```python
from build123d import *

# Parameters (mm, degrees)
SKETCH1_W           = 91.44
SKETCH1_H           = 152.4
BOSS_EXTRUDE1_DEPTH = 1.6
CUT_EXTRUDE1_REACH  = 90.878
SKETCH2_R           = 1.75
SKETCH3_W           = 91.44
SKETCH3_H           = 3
CUT_EXTRUDE2_DEPTH  = 0.0001


with BuildPart() as part:
    # Sketch1 → Boss-Extrude1 (new body)
    with BuildSketch(Plane(origin=(0, 0, 0), x_dir=(1, 0, 0), z_dir=(0, 1, 0))):
        Rectangle(SKETCH1_W, SKETCH1_H)
    extrude(amount=BOSS_EXTRUDE1_DEPTH)

    # Sketch2 → Cut-Extrude1 (cut, up to next)
    with BuildSketch(Plane(origin=(0, 1.6, 0), x_dir=(1, 0, 0), z_dir=(0, 1, 0)), mode=Mode.PRIVATE) as cut_extrude1_sk1:
        with Locations(Location((-38.22, 70.2, 0), (0, 0, 270))):
            Circle(SKETCH2_R)
    cut_extrude1_tool1 = extrude(cut_extrude1_sk1.sketch, amount=-CUT_EXTRUDE1_REACH, mode=Mode.PRIVATE) & part.part
    # Sketch2 → Cut-Extrude1 (cut, up to next)
    with BuildSketch(Plane(origin=(0, 1.6, 0), x_dir=(1, 0, 0), z_dir=(0, 1, 0)), mode=Mode.PRIVATE) as cut_extrude1_sk2:
        with Locations(Location((-33.72, -70.2, 0), (0, 0, 270))):
            Circle(SKETCH2_R)
    cut_extrude1_tool2 = extrude(cut_extrude1_sk2.sketch, amount=-CUT_EXTRUDE1_REACH, mode=Mode.PRIVATE) & part.part
    # Sketch2 → Cut-Extrude1 (cut, up to next)
    with BuildSketch(Plane(origin=(0, 1.6, 0), x_dir=(1, 0, 0), z_dir=(0, 1, 0)), mode=Mode.PRIVATE) as cut_extrude1_sk3:
        with Locations(Location((35.72, -70.2, 0), (0, 0, 270))):
            Circle(SKETCH2_R)
    cut_extrude1_tool3 = extrude(cut_extrude1_sk3.sketch, amount=-CUT_EXTRUDE1_REACH, mode=Mode.PRIVATE) & part.part
    # Sketch2 → Cut-Extrude1 (cut, up to next)
    with BuildSketch(Plane(origin=(0, 1.6, 0), x_dir=(1, 0, 0), z_dir=(0, 1, 0)), mode=Mode.PRIVATE) as cut_extrude1_sk4:
        with Locations(Location((13.78, 70.2, 0), (0, 0, 270))):
            Circle(SKETCH2_R)
    cut_extrude1_tool4 = extrude(cut_extrude1_sk4.sketch, amount=-CUT_EXTRUDE1_REACH, mode=Mode.PRIVATE) & part.part
    add(cut_extrude1_tool1.solids().sort_by_distance((-38.22, 1.6, -70.2))[0], mode=Mode.SUBTRACT)
    add(cut_extrude1_tool2.solids().sort_by_distance((-33.72, 1.6, 70.2))[0], mode=Mode.SUBTRACT)
    add(cut_extrude1_tool3.solids().sort_by_distance((35.72, 1.6, 70.2))[0], mode=Mode.SUBTRACT)
    add(cut_extrude1_tool4.solids().sort_by_distance((13.78, 1.6, -70.2))[0], mode=Mode.SUBTRACT)

    # Sketch3 → Cut-Extrude2 (cut)
    with BuildSketch(Plane(origin=(0, 1.6, 0), x_dir=(1, 0, 0), z_dir=(0, 1, 0))):
        with Locations((0, 74.7)):
            Rectangle(SKETCH3_W, SKETCH3_H)
        with Locations((0, -74.7)):
            Rectangle(SKETCH3_W, SKETCH3_H)
    extrude(amount=-CUT_EXTRUDE2_DEPTH, mode=Mode.SUBTRACT)


solid = part.part
```
Source: CAD feature listing. Evaluate the final solid. Frame: model axes, mm. Coordinates: 2 decimals unless noted, no trailing zeros. Write each loop counter-clockwise with the first axis right and the second up, starting at its lowest first coordinate (ties: lowest second). Pieces come first, ordered by that corner, then holes. Notation, with made-up numbers: (72, 83) - (108, 83) arc R23 ccw to (108, 102) - close; hole circle Ø1 at (3, 46). An arc over 180 degrees is marked (long way). Answer as a JSON object with one key per item and string values.
Q1. Draft query along Z for faces 1 (the flat face through (-1, 1.6, 75)), 2 (the cylindrical face through (13.86, 0.81, -71.95)), 3 (the cylindrical face through (34.01, 0.81, 69.82)). Return one class per face: released by +Z, released by -Z, zero draft, split by the parting line, or undercut.
Ans:
{"face 1": "zero draft", "face 2": "undercut", "face 3": "undercut"}
Q2. Section query B-B, the plane z = 70.2. Output: boundary loops of the cut face in (x, y), plus the area to 3 significant figures.
Ans:
{"outline": "(-45.72, 0) - (-35.47, 0) - (-35.47, 1.6) - (-45.72, 1.6) - close; (-31.97, 0) - (33.97, 0) - (33.97, 1.6) - (-31.97, 1.6) - close; (37.47, 0) - (45.72, 0) - (45.72, 1.6) - (37.47, 1.6) - close", "area": "135 mm2"}
Q3. First-contact query: pin 1 Ø4 at (x, z) = (13.78, -70.2) entering from +Y; pin 2 Ø3 at (x, z) = (-33.72, 70.2) entering from -Y. Flat tips, straight axial feed; report the tip coordinate or a pass-through.
Ans:
{"pin 1": "stops at y = 1.6", "pin 2": "passes through"}
Q4. Material intervals for line 1 (X direction, y = 0.6, z = 70.2); line 2 (X direction, y = 0.95, z = -70.2); line 3 (Z direction, x = -38, y = 0.9), sorted ascending. Write a range as [from, to].
Ans:
{"line 1": "x = [-45.72, -35.47], [-31.97, 33.97], [37.47, 45.72]", "line 2": "x = [-45.72, -39.97], [-36.47, 12.03], [15.53, 45.72]", "line 3": "z = [-76.2, -71.94], [-68.46, 76.2]"}
